Check sheet for the drawn part. Datum: minimum x, y, z corner. Units: mm. A direction names the side the tool comes from. Give positions to 0.01 mm unless a question says otherwise; leave off trailing zeros. Loops run counter-clockwise (first coordinate to the right, second up) from the corner with the lowest first, then second, coordinate; pieces in that order, holes last. Notation, with made-up numbers: (78.5, 87.5) - (105.5, 87.5) arc R17 ccw to (105.5, 95.5) - close; hole circle Ø7 at (-30, 7). An arc over 180 degrees is marked (long way). Answer in a Markdown table with one row per item.
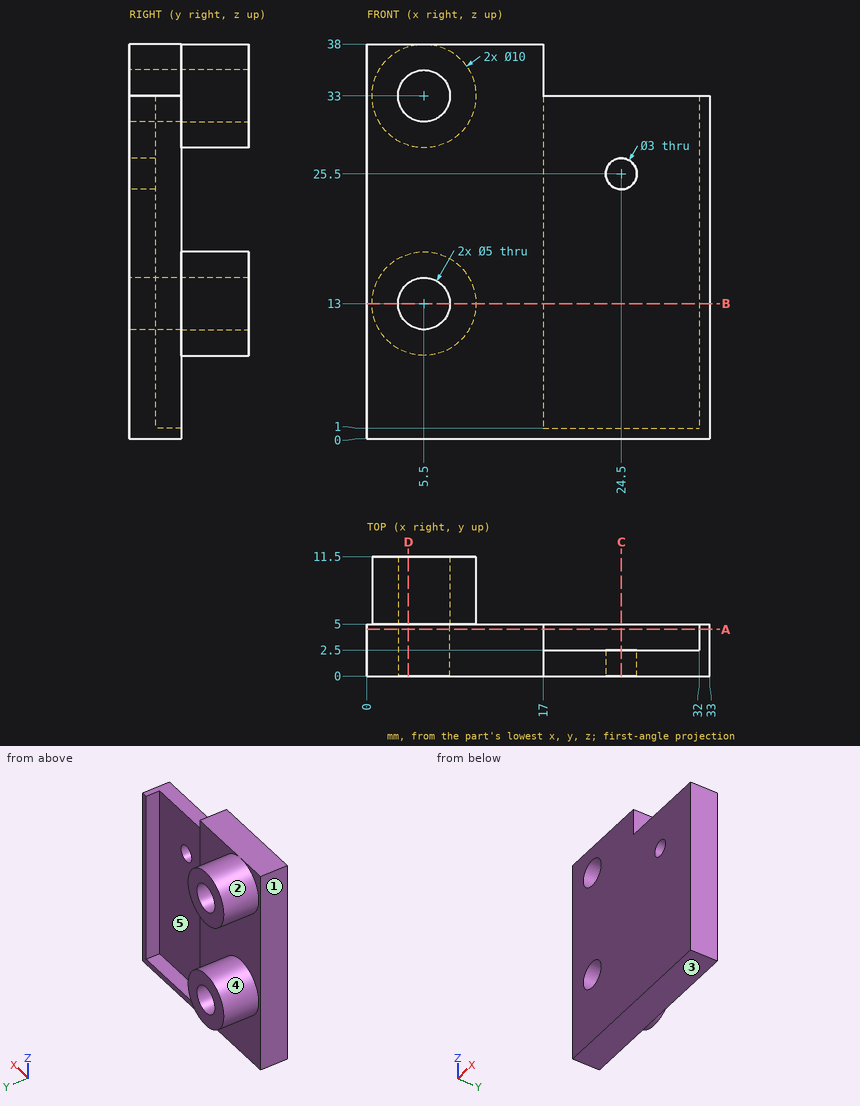
Q1. Sectioned sample at B-B (z = 13). Record the cut outline in (x, y), and give its area (3 significant figures).
Completed:
| item | result |
|---|---|
| outline | (0, 0) - (3, 0) - (3, 11.5) - (0.5, 11.5) - (0.5, 5) - (0, 5) - close; (8, 0) - (33, 0) - (33, 5) - (32, 5) - (32, 2.5) - (17, 2.5) - (17, 5) - (10.5, 5) - (10.5, 11.5) - (8, 11.5) - close |
| area | 135 mm^2 |
Q2. Tool access check on the marked faces 1 and 2. Record the directions out of +Z, -Z, +X, -X, +Y, -Y that give a thin tool (end or side, any length) a straight path to the whole face; none if there is none.
Completed:
| item | result |
|---|---|
| face 1 | +Z, -Z, -X, +Y, -Y |
| face 2 | +Y |
Q3. Draft check along X on the marked faces 3, 4 and 5. Enter one of: +X half, -X half, draft (parallel to the pull), parting line (faces both ways), or undercut.
Completed:
| item | result |
|---|---|
| face 3 | draft |
| face 4 | parting line |
| face 5 | undercut |
Q4. Thickness scan on line 1 (Z direction, x = 5.5, y = 4.5); line 2 (X direction, y = 4.25, z = 13); line 3 (X direction, y = 3.5, z = 26.5). Record the ranges inside material, lowest first.
Completed:
| item | result |
|---|---|
| line 1 | 0 to 10.5, 15.5 to 30.5, 35.5 to 38 |
| line 2 | 0 to 3, 8 to 17, 32 to 33 |
| line 3 | 0 to 17, 32 to 33 |
Q5. Sectioned sample at A-A (y = 4.5). Record the cut outline in (x, z), and give its area (3 significant figures).
Completed:
| item | result |
|---|---|
| outline | (0, 0) - (33, 0) - (33, 33) - (32, 33) - (32, 1) - (17, 1) - (17, 38) - (0, 38) - close; hole circle Ø5 at (5.5, 13); hole circle Ø5 at (5.5, 33) |
| area | 655 mm^2 |
Q6. Sectioned sample at D-D (x = 4). Record the cut outline in (y, z).
Completed:
| item | result |
|---|---|
| outline | (0, 0) - (5, 0) - (5, 8.23) - (11.5, 8.23) - (11.5, 11) - (0, 11) - close; (0, 15) - (11.5, 15) - (11.5, 17.77) - (5, 17.77) - (5, 28.23) - (11.5, 28.23) - (11.5, 31) - (0, 31) - close; (0, 35) - (11.5, 35) - (11.5, 37.77) - (5, 37.77) - (5, 38) - (0, 38) - close |
Q7. Sectioned sample at C-C (x = 24.5). Record the cut outline in (y, z), and give its area (3 significant figures).
Completed:
| item | result |
|---|---|
| outline | (0, 0) - (5, 0) - (5, 1) - (2.5, 1) - (2.5, 24) - (0, 24) - close; (0, 27) - (2.5, 27) - (2.5, 33) - (0, 33) - close |
| area | 77.5 mm^2 |
Q8. Go/stop test with flat-tipped pins: P1, Ø5, axis at x = 14.5, z = 20.5, coming from the -Y side; P2, Ø12, axis at x = 27, z = 22.5, coming from the +Y side; P3, Ø8, axis at x = 26, z = 5.5, coming from the +Y side; P4, Ø3, axis at x = 4, y = 7, coming from the -Z side. Record where each tip stops, or that it passes through.
Completed:
| item | result |
|---|---|
| P1 | y = 0 |
| P2 | y = 5 |
| P3 | y = 2.5 |
| P4 | z = 8 |
